For this review, take the finished solid that the model builds, in its own axes (mm). Face numbers are marked on the shaded views. A direction names the side the tool comes from. Round coordinates to 2 decimals unless told otherwise and drop trailing zeros. Order: outer loops, then holes, each group sorted by start corner. A loop starts at its lowest first (then second) coordinate and runs counter-clockwise, first axis right, second up. Notation, with made-up numbers: M -5,50.25 L 16,50.25 A28 cw 16,81.25 Z; hole C -27,-1.5 d6. An arc over 180 degrees is marked long. Answer as a JSON object with one key per item and string values.
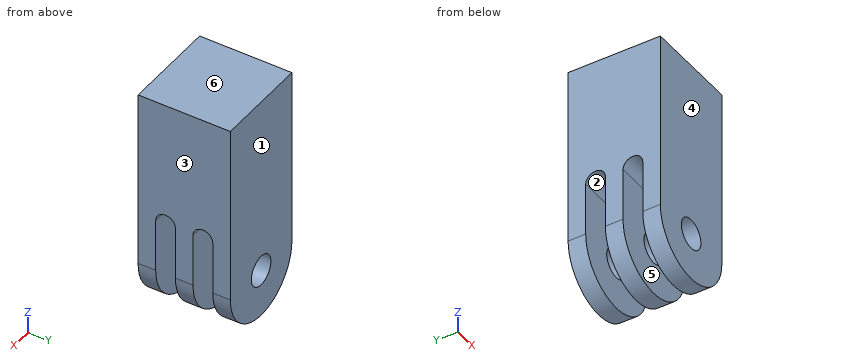
from build123d import *

# Parameters (mm, degrees)
F0_R          = 2.54
F1_DEPTH      = 7.7216
F1_DEPTH_BACK = 7.7216
F3_DEPTH      = 8.002
F3_DEPTH_BACK = 8.002


with BuildPart() as f1:
    # F0 (on Front) → F1 (new body, two sides)
    with BuildSketch(Plane.XZ) as f1_sk:
        with BuildLine():
            Line((-8.001, 30.099), (-8.001, 0))
            ThreePointArc((-8.001, 0), (0, -8.001), (8.001, 0))
            Line((8.001, 0), (8.001, 30.099))
            Line((8.001, 30.099), (-8.001, 30.099))
        make_face()
        Circle(F0_R, mode=Mode.SUBTRACT)
    extrude(amount=F1_DEPTH)
    extrude(f1_sk.sketch, amount=-F1_DEPTH_BACK)

    # F2 (on Right) → F3 (cut, two sides)
    with BuildSketch(Plane.YZ) as f3_sk:
        with BuildLine():
            Line((1.4732, 8.89), (1.4732, -10.7479624593))
            Line((1.4732, -10.7479624593), (4.7752, -10.7479624593))
            Line((4.7752, -10.7479624593), (4.7752, 8.89))
            ThreePointArc((4.7752, 8.89), (3.1242, 10.541), (1.4732, 8.89))
        make_face()
        with BuildLine():
            Line((-4.7752, 8.89), (-4.7752, -10.7479624593))
            Line((-4.7752, -10.7479624593), (-1.4732, -10.7479624593))
            Line((-1.4732, -10.7479624593), (-1.4732, 8.89))
            ThreePointArc((-1.4732, 8.89), (-3.1242, 10.541), (-4.7752, 8.89))
        make_face()
    extrude(amount=-F3_DEPTH, mode=Mode.SUBTRACT)
    extrude(f3_sk.sketch, amount=F3_DEPTH_BACK, mode=Mode.SUBTRACT)


solid = f1.part
1) For L1, parallel to Y at x = -4, z = 6; L2, parallel to X at y = 6.4, z = 0; L3, parallel to Z at x = 0, y = -5.8, list the stretches that pass through material, from the lowest coordinate up.
Geometry check:
{"L1": "y = -7.72 to -4.78, -1.47 to 1.47, 4.78 to 7.72", "L2": "x = -8 to -2.54, 2.54 to 8", "L3": "z = -8 to -2.54, 2.54 to 30.1"}
2) Mouldability with a two-part tool opening along Y and no side actions: class the marked faces 1, 2, 3 and 4 as +Y half, -Y half, draft (parallel to the pull), parting line (faces both ways), or undercut.
Geometry check:
{"face 1": "+Y half", "face 2": "undercut", "face 3": "draft", "face 4": "-Y half"}
3) Insertion check: P1, Ø3, axis at x = 0, z = 0, coming from the -Y side; P2, Ø2, axis at x = -1.5, y = 3, coming from the -Z side. Each pin has a flat end and moves straight along its axis. Give the tip position at first contact, or say it passes through.
Geometry check:
{"P1": "passes through", "P2": "stops at z = 10.1"}
4) Add section B-B on z = 4.5. State the section outline as (x, y) points, and give its area (3 significant figures).
Geometry check:
{"outline": "M -8,-7.72 L 8,-7.72 L 8,-4.78 L -8,-4.78 Z; M -8,-1.47 L 8,-1.47 L 8,1.47 L -8,1.47 Z; M -8,4.78 L 8,4.78 L 8,7.72 L -8,7.72 Z", "area": "141 mm²"}
5) Add section D-D on x = 4.5. State the section outline as (y, z) points.
Geometry check:
{"outline": "M -7.72,-6.62 L -4.78,-6.62 L -4.78,8.89 A1.65 cw -1.47,8.89 L -1.47,-6.62 L 1.47,-6.62 L 1.47,8.89 A1.65 cw 4.78,8.89 L 4.78,-6.62 L 7.72,-6.62 L 7.72,30.1 L -7.72,30.1 Z"}
6) Add section C-C on y = -1. State the section outline as (x, z) points.
Geometry check:
{"outline": "M -8,0 A8 ccw 8,0 L 8,30.1 L -8,30.1 Z; hole C 0,0 d5.08"}
7) Machinability: for the marked faces 5 and 6, which of the approach directions +Z, -Z, +X, -X, +Y, -Y give a long, thin tool a straight path to every point of the face, cutting with its end or side? Answer none if there is none.
Geometry check:
{"face 5": "-Z, +X, -X", "face 6": "+Z, +X, -X, +Y, -Y"}
8) Add section A-A on x = 0. State the section outline as (y, z) points, and give its area (3 significant figures).
Geometry check:
{"outline": "M -7.72,-8 L -4.78,-8 L -4.78,-2.54 L -7.72,-2.54 Z; M -7.72,2.54 L -4.78,2.54 L -4.78,8.89 A1.65 cw -1.47,8.89 L -1.47,2.54 L 1.47,2.54 L 1.47,8.89 A1.65 cw 4.78,8.89 L 4.78,2.54 L 7.72,2.54 L 7.72,30.1 L -7.72,30.1 Z; M -1.47,-8 L 1.47,-8 L 1.47,-2.54 L -1.47,-2.54 Z; M 4.78,-8 L 7.72,-8 L 7.72,-2.54 L 4.78,-2.54 Z", "area": "423 mm²"}
